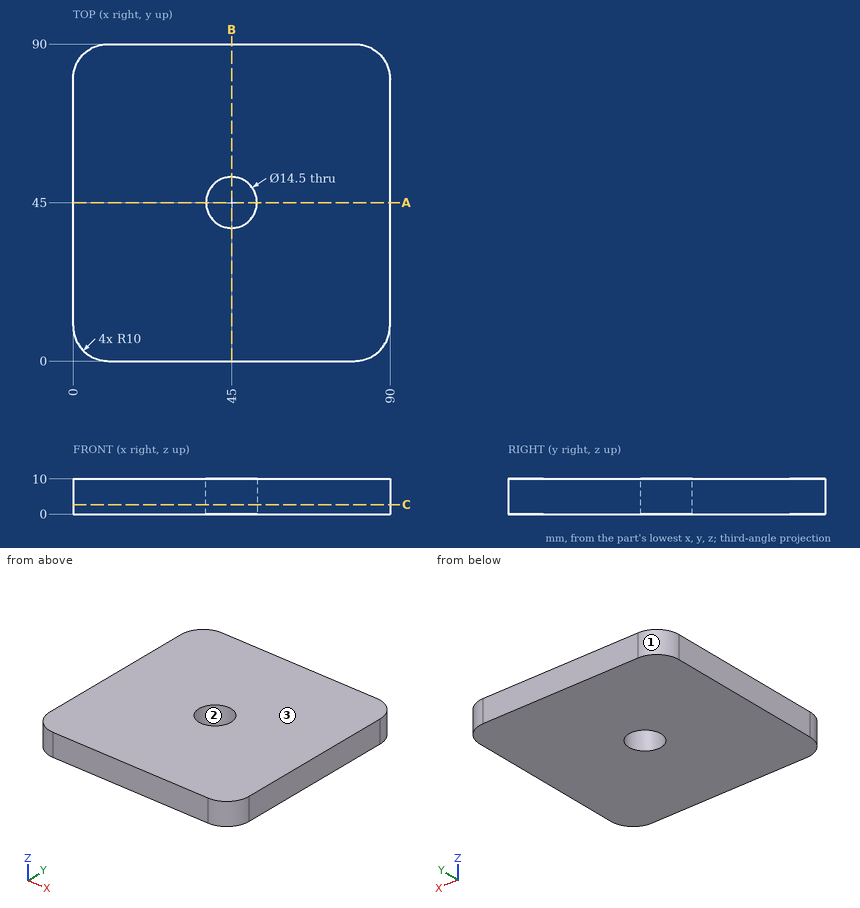
Could you check a few things on this drawing? It's one solid part, dimensions in mm from its lowest x, y, z. Give positions to 0.01 mm unless a question says otherwise; leave off trailing zeros. Write each loop counter-clockwise with the first axis right and the second up, starting at its lowest first coordinate (ties: lowest second). Pieces come first, ordered by that corner, then holes. Notation, with made-up numbers: (12, 76.5) -> (71, 76.5) arc R18 cw to (71, 96.5) -> close; hole circle Ø5 at (-25, -38.5). An arc over 180 degrees is marked (long way). Answer as a JSON object with one key per item and string values.
Q1. We'd pull the mould along X, two halves only. Please class the marked faces 1, 2 and 3: released by +X, released by -X, zero draft, split by the parting line, or undercut.
Taken from the geometry:
{"face 1": "released by -X", "face 2": "undercut", "face 3": "zero draft"}
Q2. Suppose I cut it at A-A on y = 45. Write out the boundary of the cut face in (x, z), then the cut area to 3 significant figures.
Taken from the geometry:
{"outline": "(0, 0) -> (37.75, 0) -> (37.75, 10) -> (0, 10) -> close; (52.25, 0) -> (90, 0) -> (90, 10) -> (52.25, 10) -> close", "area": "755 mm²"}
Q3. Suppose I cut it at C-C on z = 2.75. Write out the boundary of the cut face in (x, y).
Taken from the geometry:
{"outline": "(0, 10) arc R10 ccw to (10, 0) -> (80, 0) arc R10 ccw to (90, 10) -> (90, 80) arc R10 ccw to (80, 90) -> (10, 90) arc R10 ccw to (0, 80) -> close; hole circle Ø14.5 at (45, 45)"}
Q4. Please list where these lines run through material, in increasing order: L1, parallel to Y at x = 45, z = 2.25; L2, parallel to Y at x = 38.5, z = 4.5; L3, parallel to X at y = 41, z = 8.75.
Taken from the geometry:
{"L1": "y = 0 to 37.75, 52.25 to 90", "L2": "y = 0 to 41.79, 48.21 to 90", "L3": "x = 0 to 38.95, 51.05 to 90"}
